from build123d import *

# Parameters (mm, degrees)
EXTRUDE_1_DEPTH     = 50
EXTRUDE_3_DEPTH     = 5
EXTRUDE_4_DEPTH     = 1
CUT_EXTRUDE_START   = -27
CUT_EXTRUDE_2_DEPTH = 27
RIB_1_REACH         = 82.675
SKETCH_8_WALL_W     = 167.172938794
SKETCH_8_WALL_H     = 5


with BuildPart() as part:
    # 草图1 → 凸台-拉伸1 (new, symmetric)
    with BuildSketch(Plane.XY):
        with BuildLine():
            Line((-22, 0), (-20, 0))
            ThreePointArc((-20, 0), (0, 20), (20, 0))
            Line((20, 0), (22, 0))
            ThreePointArc((22, 0), (0, 22), (-22, 0))
        make_face()
    extrude(amount=EXTRUDE_1_DEPTH, both=True)

    # 草图2 → 凸台-拉伸3 (add)
    with BuildSketch(Plane.XY.offset(21)):
        with BuildLine():
            Line((-24.585593375, 15.877042923), (-35.01647279, 3.949870066))
            ThreePointArc((-35.01647279, 3.949870066), (-33.703063099, -5.073498476), (-24.991803279, -2.379026877))
            Line((-24.991803279, -2.379026877), (-20.196721311, 8.723098547))
            ThreePointArc((-20.196721311, 8.723098547), (-19.222070856, 10.701027615), (-18.054320126, 12.571456749))
            ThreePointArc((-18.054320126, 12.571456749), (-20.036220369, 16.760693495), (-24.585593375, 15.877042923))
        make_face()
        with BuildLine():
            Line((-33.627552512, 2.493675056), (-23.696783161, 14.948787263))
            ThreePointArc((-23.696783161, 14.948787263), (-20.37363516, 15.482465408), (-19.530762331, 12.223985641))
            Line((-19.530762331, 12.223985641), (-26.961919184, -1.866007539))
            ThreePointArc((-26.961919184, -1.866007539), (-32.68948429, -3.347560088), (-33.627552512, 2.493675056))
        make_face(mode=Mode.SUBTRACT)
    extrude(amount=-EXTRUDE_3_DEPTH)

    # 草图3 → 凸台-拉伸4 (add)
    with BuildSketch(Plane.XY.offset(21)):
        with BuildLine():
            Line((-23.696783161, 14.948787263), (-33.627552512, 2.493675056))
            ThreePointArc((-33.627552512, 2.493675056), (-32.68948429, -3.347560088), (-26.961919184, -1.866007539))
            Line((-26.961919184, -1.866007539), (-19.530762331, 12.223985641))
            ThreePointArc((-19.530762331, 12.223985641), (-20.37363516, 15.482465408), (-23.696783161, 14.948787263))
        make_face()
    extrude(amount=-EXTRUDE_4_DEPTH)

    # 草图6 → 切除-拉伸2 (cut)
    with BuildSketch(Plane(origin=(0, 0, -18), x_dir=(-1, 0, 0), z_dir=(0, 0, -1)).offset(CUT_EXTRUDE_START)):
        with BuildLine():
            Line((20, 0), (22, 0))
            ThreePointArc((22, 0), (21.478512157, 4.761671507), (19.938771315, 9.297601758))
            Line((19.938771315, 9.297601758), (18.126155741, 8.452365235))
            ThreePointArc((18.126155741, 8.452365235), (19.525920142, 4.328792279), (20, 0))
        make_face()
    extrude(amount=CUT_EXTRUDE_2_DEPTH, mode=Mode.SUBTRACT)

    # 草图8 wall → 筋1 (add, up to next)
    with BuildSketch(Plane(origin=(-23.495901639, -1.189513438, 18.5), x_dir=(0.782705129214, 0.622392706177, 0), z_dir=(-0.622392706177, 0.782705129214, 0)), mode=Mode.PRIVATE) as rib_1_sk1:
        Rectangle(SKETCH_8_WALL_W, SKETCH_8_WALL_H)
    rib_1_tool1 = extrude(rib_1_sk1.sketch, amount=RIB_1_REACH, mode=Mode.PRIVATE) - part.part
    add(rib_1_tool1.solids().sort_by_distance((-23.495901639, -1.189513438, 18.5))[0])


solid = part.part
Input: part model. Units: mm. Frame: model coordinates. A direction names the side the tool comes from. Round coordinates to 2 decimals unless told otherwise and drop trailing zeros. Order: outer loops, then holes, each group sorted by start corner. A loop starts at its lowest first (then second) coordinate and runs counter-clockwise, first axis right, second up. Notation, with made-up numbers: (-6.5, -22) - (29.5, -22) arc R22 ccw to (29.5, -2) - close; hole circle Ø10 at (83, 66.5). An arc over 180 degrees is marked (long way). Answer as a JSON object with one key per item and string values. Group by question number.
(1) Draft query along X for faces 6 (the face through (-23.52, -1.21, 18.46)), 7 (the face through (-19.045, 8.881, -4.311)), 8 (the face through (-32.61, -3.4, 18.03)). Return one class per face: released by +X, released by -X, zero draft, split by the parting line, or undercut.
(2) Pin query (flat end, axial travel): P1, Ø7, axis at x = -30.5, y = 0, coming from the -Z side; P2, Ø1.6, axis at x = 21.5, z = 3, coming from the -Y side; P3, Ø6, axis at x = -12, z = -22, coming from the -Y side. Return the tip coordinate at first contact, or that it passes through.
(3) Cut plane B-B (z = 34). Return loops of the section in (x, y).
(4) Material intervals for probe 1 along Z at (x, y) = (-21, 0.5); probe 2 along X at (y, z) = (8.5, 19.5); probe 3 along Y at (x, z) = (-30.5, 18.5), sorted ascending. Write a range as from..to.
(5) Cut plane C-C (z = -17). Return loops of the section in (x, y).
(6) Reachability of faces 1 (the face through (-3, 20, -50)), 2 (the face through (-21, 0, 30)), 3 (the face through (-20, 5, -18)), 4 (the face through (-20.4, 15.5, 18)), 5 (the face through (-26, 5, 21)) from +Z, -Z, +X, -X, +Y, -Y: full face, straight path, thin tool, end or side. Return the list, or none.
(7) Cut plane A-A (x = -29.5). Return loops of the section in (y, z), then the cut area to 3 significant figures.
Here are the results:
{
 "1": {"face 6": "released by +X", "face 7": "released by -X", "face 8": "undercut"},
 "2": {"P1": "stops at z = 20", "P2": "stops at y = 0", "P3": "stops at y = 13.23"},
 "3": {"outline": "(-22, 0) - (-20, 0) arc R20 cw to (20, 0) - (22, 0) arc R22 ccw to start"},
 "4": {"probe 1": "z = -50..-18, 9..50", "probe 2": "x = -31.04..-28.84, -21.49..-18.1, 18.1..20.29", "probe 3": "y = -6..-4, 6.42..9.11"},
 "5": {"outline": "(-19.94, 9.3) - (-18.13, 8.45) arc R20 cw to (20, 0) - (22, 0) arc R22 ccw to start"},
 "6": {"face 1": "-Z, +X, -X, +Y, -Y", "face 2": "+Z, -Z, +X, -Y", "face 3": "-X, -Y", "face 4": "-Z", "face 5": "+Z, -X, +Y"},
 "7": {"outline": "(-5.92, 16) - (-3.87, 16) - (-3.87, 20) - (7.67, 20) - (7.67, 16) - (10.26, 16) - (10.26, 21) - (-5.92, 21) - close", "area": "34.7 mm^2"}
}
